Input: part model. Units: mm. Frame: model coordinates. A direction names the side the tool comes from. Coordinates: 2 decimals unless noted, no trailing zeros. Write each loop counter-clockwise with the first axis right and the second up, starting at its lowest first coordinate (ties: lowest second). Pieces come first, ordered by that corner, then holes. Notation, with made-up numbers: (29, -22.75) - (82, -22.75) arc R9 ccw to (82, -13.75) - close; hole circle Ø1 at (47, -11.75). An arc over 180 degrees is marked (long way). Put each result on its own line as item: value. Start each with the question number.
1. Cut plane D-D, the plane x = -5. Return loops of the section in (y, z) (3 decimals), and give its area (3 significant figures).
2. Cut plane C-C, the plane z = -98. Return loops of the section in (x, y).
3. Pin query (flat end, axial travel): pin 1 (10 mm diameter, centred on x = 2.5, z = -16, fed in from +Y); pin 2 (0.8 mm diameter, centred on x = -20.5, z = 5.5, fed in from +Y); pin 3 (0.8 mm diameter, centred on x = 20, z = -21, fed in from -Y). Return the tip coordinate at first contact, or that it passes through.
4. Pull-direction query (X, two-part tool) for faces 1 (the cylindrical face through (23.62, 7.44, 11.27)), 2 (the cylindrical face through (-13.38, -13.65, -132.91)), 3 (the flat face through (0, 21.59, -8)); classes: released by +X, released by -X, zero draft, split by the parting line, or undercut.
5. Cut plane B-B, the plane x = -14. Return loops of the section in (y, z).
6. Line query: line 1 (Z direction, x = -25, y = -12); line 2 (Z direction, x = -9, y = -11.5); line 3 (X direction, y = -9, z = 14.5). Output: solid intervals per line, ascending.
7. Access query for faces 4 (the cylindrical face through (-13.65, 13.38, -132.91)), 5 (the cylindrical face through (13.38, 13.65, -132.91)), 6 (the flat face through (-21.59, 0, -133)), 7 (the flat face through (0, -21.59, -133)), 8 (the cylindrical face through (-13.65, -13.38, -7.82)). Directions: +Z, -Z, +X, -X, +Y, -Y. A direction counts if a zero-diameter tool reaches every point of the face in a straight line with its end or side. Return the directions, or none.
from build123d import *

# Parameters (mm, degrees)
F0_R     = 24.765
F1_DEPTH = 22.86
F2_R     = 31.75
F2_R_2   = 24.765
F3_DEPTH = 101.6
F6_DEPTH = 62.23
F7_DEPTH = 63.5


# Not quite as in the source:
# - a pattern or mirror of a feature is missing from the dataset's text; its kind, count and spacing are read off the source's solid


with BuildPart() as f1:
    # F0 (on Top) → F1 (new body)
    with BuildSketch(Plane.XY):
        Circle(F0_R)
    extrude(amount=F1_DEPTH)

    # F2 (on face) → F3 (join)
    with BuildSketch(Plane(origin=(0, 0, 0), x_dir=(1, 0, 0), z_dir=(0, 0, -1))):
        Circle(F2_R)
        Circle(F2_R_2, mode=Mode.SUBTRACT)
        Circle(F2_R_2)
    extrude(amount=F3_DEPTH)

    # F5 (on face) → F6 (cut)
    with BuildSketch(Plane.XY.offset(22.86)):
        with BuildLine():
            Line((-21.59, 1.5875), (-21.59, 0))
            Line((-21.59, 0), (-21.59, -1.5875))
            Line((-21.59, -1.5875), (-19.05, -1.5875))
            ThreePointArc((-19.05, -1.5875), (-13.517075428, -13.517075428), (-1.5875, -19.05))
            Line((-1.5875, -19.05), (-1.5875, -21.59))
            Line((-1.5875, -21.59), (1.5875, -21.59))
            Line((1.5875, -21.59), (1.5875, -19.05))
            ThreePointArc((1.5875, -19.05), (13.517075428, -13.517075428), (19.05, -1.5875))
            Line((19.05, -1.5875), (21.59, -1.5875))
            Line((21.59, -1.5875), (21.59, 0))
            Line((21.59, 0), (21.59, 1.5875))
            Line((21.59, 1.5875), (19.05, 1.5875))
            ThreePointArc((19.05, 1.5875), (13.517075428, 13.517075428), (1.5875, 19.05))
            Line((1.5875, 19.05), (1.5875, 21.59))
            Line((1.5875, 21.59), (-1.5875, 21.59))
            Line((-1.5875, 21.59), (-1.5875, 19.05))
            ThreePointArc((-1.5875, 19.05), (-13.517075428, 13.517075428), (-19.05, 1.5875))
            Line((-19.05, 1.5875), (-21.59, 1.5875))
        make_face()
    extrude(amount=-F6_DEPTH, mode=Mode.SUBTRACT)

    # F4 (on face) → F7 (join)
    with BuildSketch(Plane(origin=(0, 0, -101.6), x_dir=(1, 0, 0), z_dir=(0, 0, -1))):
        with BuildLine():
            Line((-21.59, 1.5875), (-21.59, 0))
            Line((-21.59, 0), (-21.59, -1.5875))
            Line((-21.59, -1.5875), (-19.05, -1.5875))
            ThreePointArc((-19.05, -1.5875), (-13.517075428, -13.517075428), (-1.5875, -19.05))
            Line((-1.5875, -19.05), (-1.5875, -21.59))
            Line((-1.5875, -21.59), (1.5875, -21.59))
            Line((1.5875, -21.59), (1.5875, -19.05))
            ThreePointArc((1.5875, -19.05), (13.517075428, -13.517075428), (19.05, -1.5875))
            Line((19.05, -1.5875), (21.59, -1.5875))
            Line((21.59, -1.5875), (21.59, 0))
            Line((21.59, 0), (21.59, 1.5875))
            Line((21.59, 1.5875), (19.05, 1.5875))
            ThreePointArc((19.05, 1.5875), (13.517075428, 13.517075428), (1.5875, 19.05))
            Line((1.5875, 19.05), (1.5875, 21.59))
            Line((1.5875, 21.59), (-1.5875, 21.59))
            Line((-1.5875, 21.59), (-1.5875, 19.05))
            ThreePointArc((-1.5875, 19.05), (-13.517075428, 13.517075428), (-19.05, 1.5875))
            Line((-19.05, 1.5875), (-21.59, 1.5875))
        make_face()
    f7 = extrude(amount=F7_DEPTH)

    # F7_copies: F7 across plane
    add(f7.mirror(Plane.XY.offset(-102.235)))


solid = f1.part
Report:
1. outline: (-31.354, -101.6) - (-18.451, -101.6) - (-18.451, -165.1) - (18.451, -165.1) - (18.451, -101.6) - (31.354, -101.6) - (31.354, 0) - (24.255, 0) - (24.255, 22.86) - (18.451, 22.86) - (18.451, -39.37) - (-18.451, -39.37) - (-18.451, 22.86) - (-24.255, 22.86) - (-24.255, 0) - (-31.354, 0) - close
1. area: 7,530 mm^2
2. outline: circle Ø63.5 at (0, 0)
3. pin 1: stops at y = 31.75
3. pin 2: stops at y = 14.47
3. pin 3: stops at y = -24.98
4. face 1: split by the parting line
4. face 2: released by -X
4. face 3: undercut
5. outline: (-28.5, -101.6) - (-13.02, -101.6) - (-13.02, -165.1) - (13.02, -165.1) - (13.02, -101.6) - (28.5, -101.6) - (28.5, 0) - (20.43, 0) - (20.43, 22.86) - (13.02, 22.86) - (13.02, -39.37) - (-13.02, -39.37) - (-13.02, 22.86) - (-20.43, 22.86) - (-20.43, 0) - (-28.5, 0) - close
6. line 1: z = -101.6 to 0
6. line 2: z = -165.1 to -39.37
6. line 3: x = -23.07 to -16.86, 16.86 to 23.07
7. face 4: -Z, -X, +Y
7. face 5: -Z, +X, +Y
7. face 6: -Z, -X, +Y, -Y
7. face 7: -Z, +X, -X, -Y
7. face 8: +Z
